Source: CAD feature listing. Evaluate the final solid. Frame: model axes, mm. A direction names the side the tool comes from. Give positions to 0.01 mm unless a question says otherwise; leave off trailing zeros. Loops run counter-clockwise (first coordinate to the right, second up) from the corner with the lowest first, then second, coordinate; pieces in that order, holes last.
from build123d import *

# Parameters (mm, degrees)
F0_W     = 127
F0_H     = 12.7
F1_DEPTH = 25.4
F2_R     = 3.9243
F3_DEPTH = 6.35
F4_W     = 114.3
F4_H     = 9.2964
F5_DEPTH = 3.175


with BuildPart() as f1:
    # F0 (on Front) → F1 (new body)
    with BuildSketch(Plane.XZ):
        Rectangle(F0_W, F0_H)
    extrude(amount=F1_DEPTH)

    # F2 (on face) → F3 (cut)
    with BuildSketch(Plane(origin=(0, 0, 0), x_dir=(-1, 0, 0), z_dir=(0, 1, 0))):
        with Locations((40.321597, 0)):
            Circle(F2_R)
        with Locations((-52.069283, 0)):
            Circle(F2_R)
        with Locations((-40.520423, 0)):
            Circle(F2_R)
        with Locations((-28.971563, 0)):
            Circle(F2_R)
        with Locations((-17.422703, 0)):
            Circle(F2_R)
        with Locations((-5.873843, 0)):
            Circle(F2_R)
        with Locations((5.675017, 0)):
            Circle(F2_R)
        with Locations((17.223877, 0)):
            Circle(F2_R)
        with Locations((28.772737, 0)):
            Circle(F2_R)
        with Locations((51.870457, 0)):
            Circle(F2_R)
    extrude(amount=-F3_DEPTH, mode=Mode.SUBTRACT)

    # F4 (on face) → F5 (cut)
    with BuildSketch(Plane.XZ.offset(25.4)):
        Rectangle(F4_W, F4_H)
    extrude(amount=-F5_DEPTH, mode=Mode.SUBTRACT)


solid = f1.part
1) Reachability of faces 4 (the flat face through (41, -6.35, 0)), 5 (the flat face through (-1, -22.225, 0)), 6 (the flat face through (-1, 0, 0)) from +Z, -Z, +X, -X, +Y, -Y: full face, straight path, thin tool, end or side. Return the list, or none.
Checks:
face 4: +Y
face 5: -Y
face 6: +Z, -Z, +X, -X, +Y
2) Cut plane B-B (y = -2.5). State how many separate pieces and enclosed holes the cut face has, and give its area (3 significant figures).
Checks:
separate pieces: 1
enclosed holes: 10
area: 1,130 mm2
3) Pull-direction query (X, two-part tool) for faces 1 (the flat face through (-1, -13, 6.35)), 2 (the cylindrical face through (-20.85, -3.13, -1.5)), 3 (the flat face through (63.5, -13, 0)); classes: released by +X, released by -X, zero draft, split by the parting line, or undercut.
Checks:
face 1: zero draft
face 2: undercut
face 3: released by +X
4) Cut plane C-C (x = 38.5). Return loops of the section in (y, z) (3 decimals).
Checks:
outline: (-25.4, -6.35) - (0, -6.35) - (0, -3.364) - (-6.35, -3.364) - (-6.35, 3.364) - (0, 3.364) - (0, 6.35) - (-25.4, 6.35) - (-25.4, 4.648) - (-22.225, 4.648) - (-22.225, -4.648) - (-25.4, -4.648) - close
5) Cut plane D-D (x = -52). Return loops of the section in (y, z) (3 decimals).
Checks:
outline: (-25.4, -6.35) - (0, -6.35) - (0, -3.922) - (-6.35, -3.922) - (-6.35, 3.922) - (0, 3.922) - (0, 6.35) - (-25.4, 6.35) - (-25.4, 4.648) - (-22.225, 4.648) - (-22.225, -4.648) - (-25.4, -4.648) - close
6) Ray query, probe 1 along Z at (x, y) = (10.5, -23.5); probe 2 along Y at (x, z) = (23, 2.5) (3 decimals); probe 3 along Z at (x, y) = (-25.5, -2.25). Return the intervals inside material, ascending.
Checks:
probe 1: z = -6.35 to -4.65, 4.65 to 6.35
probe 2: y = -22.225 to 0
probe 3: z = -6.35 to -2.17, 2.17 to 6.35
7) Contact query for flat-ended pins moving along their axis: P1, Ø6.5, axis at x = 39.5, z = -0.5, coming from the +Y side; P2, Ø4, axis at x = 7.5, z = 0.5, coming from the +Y side; P3, Ø5, axis at x = -10.5, z = -2, coming from the -Y side (3 decimals). Output: stop coordinate, or through.
Checks:
P1: stops at y = 0
P2: stops at y = -6.35
P3: stops at y = -22.225
8) Cut plane A-A (y = -23.5). Return loops of the section in (x, z), and give its area (3 significant figures).
Checks:
outline: (-63.5, -6.35) - (63.5, -6.35) - (63.5, 6.35) - (-63.5, 6.35) - close; hole (-57.15, -4.65) - (57.15, -4.65) - (57.15, 4.65) - (-57.15, 4.65) - close
area: 550 mm2
